from build123d import *

# Parameters (mm, degrees)
SKETCH_W     = 185
SKETCH_H     = 10
SKETCH001_R  = 45
PAD_DEPTH    = 40
SKETCH002_R  = 45
PAD001_DEPTH = 20


with BuildPart() as part:
    # Sketch → Revolution (revolve)
    with BuildSketch(Plane.XY):
        with Locations((92.5, 30)):
            Rectangle(SKETCH_W, SKETCH_H)
    revolve(axis=Axis((0, 0, 0), (1, 0, 0)))

    # Sketch001 → Pad (new body, symmetric)
    with BuildSketch(Plane.XY):
        Circle(SKETCH001_R)
    extrude(amount=PAD_DEPTH, both=True)

    # Sketch002 (on Face5 of Pad) → Pad001 (join)
    with BuildSketch(Plane.XY.offset(40)):
        Circle(SKETCH002_R)
    extrude(amount=PAD001_DEPTH)


solid = part.part
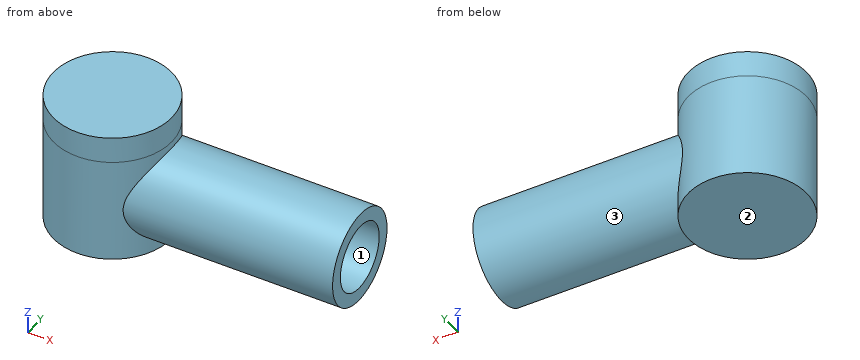
Geometry: final body of the model. Coordinates: model frame, mm. Face numbers are marked on the shaded views. Give positions to 0.01 mm unless a question says otherwise; leave off trailing zeros. Write each loop counter-clockwise with the first axis right and the second up, starting at its lowest first coordinate (ties: lowest second). Pieces come first, ordered by that corner, then holes.
(1) Cut plane D-D, the plane x = 30.5. Return loops of the section in (y, z).
(2) Mould query, pull axis Y, two halves, no side actions, for the marked faces 1, 2 and 3. Classes: released by +Y, released by -Y, zero draft, split by the parting line, or undercut.
(3) Ray query, line 1 (Z direction, x = 48, y = -1); line 2 (Y direction, x = 160.5, z = -1.5); line 3 (Y direction, x = 0.5, z = 24). Return the intervals inside material, ascending.
(4) Cut plane C-C, the plane x = 166.5. Return loops of the section in (y, z).
(5) Cut plane B-B, the plane z = 0. Return loops of the section in (x, y), then the cut area to 3 significant figures.
(6) First-contact query: P1, Ø1.5, axis at x = 109, y = 18, coming from the +Z side; P2, Ø2, axis at y = 12.5, z = 14, coming from the -X side; P3, Ø4, axis at y = 21, z = 44, coming from the -X side. Flat tips, straight axial feed; report the tip coordinate or a pass-through.
(7) Cut plane A-A, the plane y = 0. Return loops of the section in (x, z).
Values follow:
1. outline: (-33.09, -40) - (33.09, -40) - (33.09, -11.41) arc R35 ccw to (33.09, 11.41) - (33.09, 60) - (-33.09, 60) - (-33.09, 11.41) arc R35 ccw to (-33.09, -11.41) - close
2. face 1: undercut
2. face 2: zero draft
2. face 3: split by the parting line
3. line 1: z = -34.99 to -24.98, 24.98 to 34.99
3. line 2: y = -34.97 to -24.95, 24.95 to 34.97
3. line 3: y = -45 to 45
4. outline: circle Ø70 at (0, 0); hole circle Ø50 at (0, 0)
5. outline: (28.28, -35) - (185, -35) - (185, -25) - (37.42, -25) arc R45 ccw to (37.42, 25) - (185, 25) - (185, 35) - (28.28, 35) arc R45 ccw (long way) to start
5. area: 9,400 mm2
6. P1: stops at z = 30.45
6. P2: stops at x = -43.51
6. P3: stops at x = -40.79
7. outline: (-45, -40) - (45, -40) - (45, -35) - (185, -35) - (185, -25) - (45, -25) - (45, 25) - (185, 25) - (185, 35) - (45, 35) - (45, 60) - (-45, 60) - close
